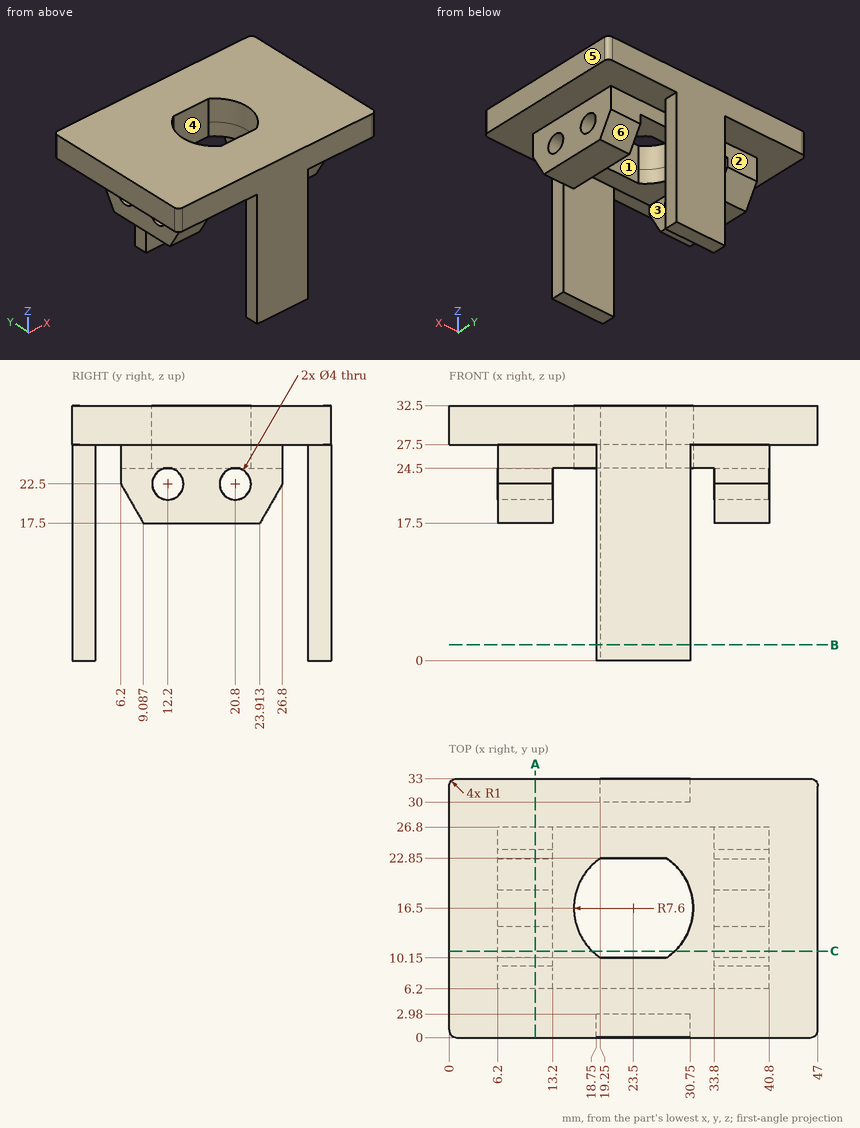
The figure shows three views and two pictorial views of one solid part (mm, origin at its lowest corner). Answer the questions. A direction names the side the tool comes from. Round coordinates to 2 decimals unless told otherwise and drop trailing zeros. Write each loop counter-clockwise with the first axis right and the second up, starting at its lowest first coordinate (ties: lowest second). Pieces come first, ordered by that corner, then holes. Notation, with made-up numbers: (1.25, 27.5) - (51.25, 27.5) arc R18 cw to (51.25, 48.5) - close; hole circle Ø2 at (37.25, -22). An arc over 180 degrees is marked (long way). Use one line per item in the form item = value. Start each with the question number.
Item 1: A cutting plane is placed at C-C (y = 11). Give the number of separate pieces and of enclosed holes in the cut face, plus the area to 3 significant figures.
Item 2: A tool of negligible diameter and unlimited length cuts with its end or side. For the marked faces 1, 2 and 3, from which of +Z, -Z, +X, -X, +Y, -Y can it reach the whole face along a straight path? Write none if from no direction.
Item 3: Determine the mould class of the marked faces 4, 5 and 6 for opening direction X: +X half, -X half, draft (parallel to the pull), parting line (faces both ways), or undercut.
Item 4: Find the intervals of material crossed by line 1 (Y direction, x = 10, z = 22.5); line 2 (X direction, y = 16.5, z = 20.5); line 3 (Z direction, x = 37, y = 12), in increasing order. Write a range as [from, to].
Item 5: A cutting plane is placed at A-A (x = 11). Write down the section's boundary in (y, z), plus the area to 3 significant figures.
Item 6: Flat-ended cylindrical pins translate along their axes: pin 1 Ø3 at (y, z) = (11.5, 23) entering from -X; pin 2 Ø3.5 at (y, z) = (12.2, 22.5) entering from +X; pin 3 Ø2.5 at (y, z) = (31.5, 12.5) entering from -X; pin 4 Ø2.5 at (y, z) = (31.5, 7.5) entering from +X. Find the tip coordinate at first contact, or state that the pin passes through.
Item 7: A cutting plane is placed at B-B (z = 2). Write down the section's boundary in (x, y).
The answers:
q1.separate_pieces = 4
q1.enclosed_holes = 0
q1.area = 308 mm^2
q2.face_1 = +Z, -Z
q2.face_2 = -Z, +X, -X
q2.face_3 = -Z, +Y, -Y
q3.face_4 = undercut
q3.face_5 = +X half
q3.face_6 = draft
q4.line_1 = [6.2, 10.2], [14.2, 18.8], [22.8, 26.8]
q4.line_2 = [6.2, 13.2], [33.8, 40.8]
q4.line_3 = [17.5, 20.51], [24.49, 32.5]
q5.outline = (0, 27.5) - (6.2, 27.5) - (6.2, 22.5) - (9.09, 17.5) - (23.91, 17.5) - (26.8, 22.5) - (26.8, 27.5) - (33, 27.5) - (33, 32.5) - (0, 32.5) - close; hole circle Ø4 at (12.2, 22.5); hole circle Ø4 at (20.8, 22.5)
q5.area = 331 mm^2
q6.pin_1 = 6.2
q6.pin_2 = through
q6.pin_3 = 19.25
q6.pin_4 = 30.75
q7.outline = (18.75, 0) - (30.75, 0) - (30.75, 2.98) - (18.75, 2.98) - close; (19.25, 30) - (30.75, 30) - (30.75, 33) - (19.25, 33) - close
